```python
from build123d import *

# Parameters (mm, degrees)
CROQUIS1_W              = 200
CROQUIS1_H              = 30
SALIENTE_EXTRUIR1_DEPTH = 3
CROQUIS2_W              = 3
CROQUIS2_H              = 20
SALIENTE_EXTRUIR2_DEPTH = 23


with BuildPart() as part:
    # Croquis1 → Saliente-Extruir1 (new body)
    with BuildSketch(Plane.XY):
        with Locations((-118.159579588, 33.85177453)):
            Rectangle(CROQUIS1_W, CROQUIS1_H)
        Polygon((-28.159579588, 43.85177453), (-28.159579588, 23.85177453), (-73.159579588, 33.85177453), align=None, mode=Mode.SUBTRACT)
        Polygon((-208.159579588, 43.85177453), (-163.159579588, 33.85177453), (-208.159579588, 23.85177453), align=None, mode=Mode.SUBTRACT)
        Polygon((-194.330262902, 43.85177453), (-156.244921245, 35.388365273), (-124.77138853, 43.85177453), align=None, mode=Mode.SUBTRACT)
        Polygon((-194.330262902, 23.85177453), (-156.244921245, 32.315183787), (-124.77138853, 23.85177453), align=None, mode=Mode.SUBTRACT)
        Polygon((-118.159579588, 40.778593045), (-149.330262902, 33.85177453), (-118.159579588, 26.924956016), (-86.988896274, 33.85177453), align=None, mode=Mode.SUBTRACT)
        Polygon((-41.988896274, 23.85177453), (-80.074237931, 32.315183787), (-112.871999428, 23.85177453), align=None, mode=Mode.SUBTRACT)
        Polygon((-41.988896274, 43.85177453), (-80.074237931, 35.388365273), (-112.871999428, 43.85177453), align=None, mode=Mode.SUBTRACT)
    extrude(amount=SALIENTE_EXTRUIR1_DEPTH)

    # Croquis2 → Saliente-Extruir2 (add)
    with BuildSketch(Plane.XY.offset(3)):
        with Locations((-216.659579588, 28.85177453)):
            Rectangle(CROQUIS2_W, CROQUIS2_H)
        with Locations((-19.659579588, 28.85177453)):
            Rectangle(CROQUIS2_W, CROQUIS2_H)
    extrude(amount=-SALIENTE_EXTRUIR2_DEPTH)


solid = part.part
```
The model under review builds one solid part; all positions refer to its coordinate system, in mm. A direction names the side the tool comes from. Coordinates: 2 decimals unless noted, no trailing zeros. Loops run counter-clockwise (first coordinate to the right, second up) from the corner with the lowest first, then second, coordinate; pieces in that order, holes last. Notation, with made-up numbers: (-36, -21.75) -> (-15, -21.75) arc R12 cw to (-15, -4.75) -> close; hole circle Ø2 at (59, 34). An arc over 180 degrees is marked (long way). Answer as CSV lines item,"result".
Item 1: For L1, parallel to X at y = 27.5, z = -4; L2, parallel to Z at x = -206, y = 24.25; L3, parallel to Y at x = -187.5, z = 1.25, list the stretches that pass through material, from the lowest coordinate up.
Results below:
L1,"x = -218.16 to -215.16, -21.16 to -18.16"
L2,"z = 0 to 3"
L3,"y = 18.85 to 23.85, 25.37 to 28.44, 39.26 to 42.33, 43.85 to 48.85"
Item 2: Take a section at C-C, the plane y = 29.5. State the section outline as (x, z) points, and give its area (3 significant figures).
Results below:
outline,"(-218.16, -20) -> (-215.16, -20) -> (-215.16, 0) -> (-208.16, 0) -> (-208.16, 3) -> (-218.16, 3) -> close; (-182.74, 0) -> (-168.91, 0) -> (-168.91, 3) -> (-182.74, 3) -> close; (-145.78, 0) -> (-129.75, 0) -> (-129.75, 3) -> (-145.78, 3) -> close; (-106.57, 0) -> (-90.98, 0) -> (-90.98, 3) -> (-106.57, 3) -> close; (-67.41, 0) -> (-53.58, 0) -> (-53.58, 3) -> (-67.41, 3) -> close; (-28.16, 0) -> (-21.16, 0) -> (-21.16, -20) -> (-18.16, -20) -> (-18.16, 3) -> (-28.16, 3) -> close"
area,"358 mm2"
Item 3: Take a section at D-D, the plane x = -185.5. State the section outline as (y, z) points.
Results below:
outline,"(18.85, 0) -> (23.85, 0) -> (23.85, 3) -> (18.85, 3) -> close; (25.81, 0) -> (28.89, 0) -> (28.89, 3) -> (25.81, 3) -> close; (38.82, 0) -> (41.89, 0) -> (41.89, 3) -> (38.82, 3) -> close; (43.85, 0) -> (48.85, 0) -> (48.85, 3) -> (43.85, 3) -> close"
Item 4: Draft analysis for pull direction X (two halves, no side actions). For faces 3 (the flat face through (-185, 29, 1)), 4 (the flat face through (-133.527, 37.364, 1.479)), 5 (the flat face through (-119, 18.852, 2)), 6 (the flat face through (-18.16, 30, -9)), state which applies: +X half, -X half, draft (parallel to the pull), parting line (faces both ways), or undercut.
Results below:
face 3,"undercut"
face 4,"undercut"
face 5,"draft"
face 6,"+X half"
Item 5: Machinability: for faces 1 (the flat face through (-215.16, 29, -10)), 2 (the flat face through (-50.975, 38.782, 1.479)), which of the approach directions +Z, -Z, +X, -X, +Y, -Y give a long, thin tool a straight path to every point of the face, cutting with its end or side? Answer none if there is none.
Results below:
face 1,"-Z, +Y, -Y"
face 2,"+Z, -Z"
Item 6: Take a section at B-B, the plane z = -13.5. State the section outline as (x, y) points.
Results below:
outline,"(-218.16, 18.85) -> (-215.16, 18.85) -> (-215.16, 38.85) -> (-218.16, 38.85) -> close; (-21.16, 18.85) -> (-18.16, 18.85) -> (-18.16, 38.85) -> (-21.16, 38.85) -> close"
Item 7: Insertion check: pin 1 (5 mm diameter, centred on y = 39.5, z = -6.5, fed in from +X); pin 2 (2.5 mm diameter, centred on x = -216.5, z = -13.5, fed in from +Y); pin 3 (15 mm diameter, centred on x = -124.5, y = 32, fed in from -Z). Each pin has a flat end and moves straight along its axis. Give the tip position at first contact, or say it passes through.
Results below:
pin 1,"stops at x = -18.16"
pin 2,"stops at y = 38.85"
pin 3,"stops at z = 0"
Item 8: Take a section at A-A, the plane x = -141. State the section outline as (y, z) points, and give its area (3 significant figures).
Results below:
outline,"(18.85, 0) -> (23.85, 0) -> (23.85, 3) -> (18.85, 3) -> close; (28.22, 0) -> (32, 0) -> (32, 3) -> (28.22, 3) -> close; (35.7, 0) -> (39.49, 0) -> (39.49, 3) -> (35.7, 3) -> close; (43.85, 0) -> (48.85, 0) -> (48.85, 3) -> (43.85, 3) -> close"
area,"52.7 mm2"
